from build123d import *

# Parameters (mm, degrees)
PAD_DEPTH       = 7
POCKET_DEPTH    = 3
SKETCH002_R     = 1.75
POCKET001_DEPTH = 7.001
FILLET_R        = 1
CHAMFER_SIZE    = 1


with BuildPart() as part:
    # Sketch → Pad (new body)
    with BuildSketch(Plane.XY):
        Polygon((0, 20), (0, 0), (20, 0), align=None)
    extrude(amount=PAD_DEPTH)

    # Sketch001 (on Face5 of Pad) → Pocket (cut)
    with BuildSketch(Plane.XY.offset(7)):
        Polygon((6, 14), (6, 6), (14, 6), align=None)
    extrude(amount=-POCKET_DEPTH, mode=Mode.SUBTRACT)

    # Sketch002 (on Face5 of Pocket) → Pocket001 (cut, through all)
    with BuildSketch(Plane.XY.offset(7)):
        with Locations((3, 3)):
            Circle(SKETCH002_R)
        with Locations((12, 3)):
            Circle(SKETCH002_R)
        with Locations((3, 12)):
            Circle(SKETCH002_R)
    extrude(amount=-POCKET001_DEPTH, mode=Mode.SUBTRACT)

    # Fillet
    fillet_edges = [part.edges().sort_by_distance(p)[0] for p in [
        (0, 0, 3.5),
        (20, 0, 3.5),
        (0, 20, 3.5),
    ]]
    fillet(fillet_edges, radius=FILLET_R)

    # Chamfer
    chamfer_edges = [part.edges().sort_by_distance(p)[0] for p in [
        (1.25, 12, 0),
        (10.25, 3, 0),
        (1.25, 3, 0),
    ]]
    chamfer(chamfer_edges, length=CHAMFER_SIZE)


solid = part.part
For this review, take the finished solid that the model builds, in its own axes (mm). A direction names the side the tool comes from. Round coordinates to 2 decimals unless told otherwise and drop trailing zeros. Write each loop counter-clockwise with the first axis right and the second up, starting at its lowest first coordinate (ties: lowest second). Pieces come first, ordered by that corner, then holes. Notation, with made-up numbers: (17.5, -40) - (22.5, -40) arc R25 cw to (22.5, -12) - close; hole circle Ø5 at (56.25, -29.5). An arc over 180 degrees is marked (long way). Use a Markdown table: item, result.
Q1. We need section A-A (y = 3). Give the boundary of the cut face in (x, z), plus the area to 3 significant figures.
Derived:
| item | result |
|---|---|
| outline | (0, 0) - (0.25, 0) - (1.25, 1) - (1.25, 7) - (0, 7) - close; (4.75, 1) - (5.75, 0) - (9.25, 0) - (10.25, 1) - (10.25, 7) - (4.75, 7) - close; (13.75, 1) - (14.75, 0) - (17, 0) - (17, 7) - (13.75, 7) - close |
| area | 68.0 mm2 |
Q2. We need section B-B (z = 3.5). Give the boundary of the cut face in (x, y), plus the area to 3 significant figures.
Derived:
| item | result |
|---|---|
| outline | (0, 1) arc R1 ccw to (1, 0) - (17.59, 0) arc R1 ccw to (18.29, 1.71) - (1.71, 18.29) arc R1 ccw to (0, 17.59) - close; hole circle Ø3.5 at (3, 3); hole circle Ø3.5 at (3, 12); hole circle Ø3.5 at (12, 3) |
| area | 168 mm2 |
Q3. Clearance check with flat-ended pins moving along their axes: pin 1 (2 mm diameter, centred on y = 11, z = 6, fed in from +X); pin 2 (3 mm diameter, centred on x = 10, z = 3, fed in from +Y); pin 3 (1 mm diameter, centred on x = 12, z = 2, fed in from +Y). State where each tip first meets the part, or that it passes through.
Derived:
| item | result |
|---|---|
| pin 1 | stops at x = 6 |
| pin 2 | stops at y = 11.5 |
| pin 3 | stops at y = 8.5 |
Q4. We need section C-C (y = 12). Give the boundary of the cut face in (x, z), plus the area to 3 significant figures.
Derived:
| item | result |
|---|---|
| outline | (0, 0) - (0.25, 0) - (1.25, 1) - (1.25, 7) - (0, 7) - close; (4.75, 1) - (5.75, 0) - (8, 0) - (8, 4) - (6, 4) - (6, 7) - (4.75, 7) - close |
| area | 24.5 mm2 |
Q5. The part is to be moulded in two halves that separate along Y. For faces 3 (the cylindrical face through (2.772, 13.735, 4.042)), 4 (the cylindrical face through (18.516, 0.633, 3.549)), 5 (the flat face through (10, 10, 3)), say which applies: pulls with the +Y half, pulls with the -Y half, needs draft (parallel to the pull), parting line crosses it, or undercut.
Derived:
| item | result |
|---|---|
| face 3 | undercut |
| face 4 | parting line crosses it |
| face 5 | pulls with the +Y half |
Q6. Wall thickness on line 1 along X through (y, z) = (1.75, 4.5); line 2 along Y through (x, z) = (12, 5.15); line 3 along Y through (x, z) = (1.5, 1.25): over which ranges is each line inside the solid? List them lowest first.
Derived:
| item | result |
|---|---|
| line 1 | x = 0 to 1.78, 4.22 to 10.78, 13.22 to 18.25 |
| line 2 | y = 0 to 1.25, 4.75 to 6 |
| line 3 | y = 0 to 2.1, 3.9 to 11.1, 12.9 to 18.45 |
Q7. Machinability: for faces 1 (the flat face through (6, 10, 6)), 2 (the flat face through (5, 5, 7)), which of the approach directions +Z, -Z, +X, -X, +Y, -Y give a long, thin tool a straight path to every point of the face, cutting with its end or side? Answer none if there is none.
Derived:
| item | result |
|---|---|
| face 1 | +Z, +X, +Y |
| face 2 | +Z, +X, -X, +Y, -Y |
